from build123d import *

# Parameters (mm, degrees)
F1_DEPTH = 40


with BuildPart() as f1:
    # F0 (on Top) → F1 (new body)
    with BuildSketch(Plane.XY):
        with BuildLine():
            Line((0, 30), (0, 0))
            Line((0, 0), (30, 0))
            ThreePointArc((30, 0), (40.606601, 4.393399), (44.999999, 15))
            Line((44.999999, 15), (44.999999, 30))
            Line((44.999999, 30), (29.999999, 44.999999))
            Line((29.999999, 44.999999), (14.999999, 44.999999))
            Line((14.999999, 44.999999), (0, 30))
        make_face()
    extrude(amount=F1_DEPTH)


solid = f1.part
Build history of the part. All positions in model axes, mm. Coordinates: 2 decimals unless noted, no trailing zeros. Order: outer loops, then holes, each group sorted by start corner. A loop starts at its lowest first (then second) coordinate and runs counter-clockwise, first axis right, second up. Notation, with made-up numbers: (34.5, -13) -> (88.5, -13) arc R23 cw to (88.5, 15) -> close; hole circle Ø7 at (79, 5.25). An arc over 180 degrees is marked (long way). One line per item, written item: value.
(1) Drop flat-ended pins along their axis: pin 1 Ø10 at (x, z) = (37.5, 33) entering from +Y; pin 2 Ø12 at (y, z) = (39, 11) entering from -X. Give the stop position or say it passes through.
Checked values:
pin 1: y = 42.5
pin 2: x = 3
(2) Slice it at A-A, the plane z = 3.5. List the corners of the cut face in (x, y).
Checked values:
outline: (0, 0) -> (30, 0) arc R15 ccw to (45, 15) -> (45, 30) -> (30, 45) -> (15, 45) -> (0, 30) -> close
(3) Probe line 1 (Y direction, x = 5, z = 29.5); line 2 (X direction, y = 6, z = 20.5); line 3 (Y direction, x = 13, z = 2). List the from-to ranges inside material, lowest first. Write a range as [from, to].
Checked values:
line 1: [0, 35]
line 2: [0, 42]
line 3: [0, 43]
(4) Slice it at B-B, the plane x = 5. List the corners of the cut face in (y, z).
Checked values:
outline: (0, 0) -> (35, 0) -> (35, 40) -> (0, 40) -> close
(5) Slice it at C-C, the plane y = 6. List the corners of the cut face in (x, z).
Checked values:
outline: (0, 0) -> (42, 0) -> (42, 40) -> (0, 40) -> close
